Verification items for the finished model (mm, model axes). A direction names the side the tool comes from. Coordinates: 2 decimals unless noted, no trailing zeros. Write each loop counter-clockwise with the first axis right and the second up, starting at its lowest first coordinate (ties: lowest second). Pieces come first, ordered by that corner, then holes. Notation, with made-up numbers: M -39.5,44.25 L -34.5,44.25 A23 cw -34.5,67.25 Z; hole C 16.5,50 d5. An arc over 180 degrees is marked long. Answer in a Markdown table with one row per item.
from build123d import *

# Parameters (mm, degrees)
BOSS_EXTRUDE2_DEPTH = 3
CUT_EXTRUDE1_REACH  = 5
SKETCH2_R           = 1
SKETCH3_W           = 5.601007624
SKETCH3_H           = 10
BOSS_EXTRUDE3_DEPTH = 8
CHAMFER1_SIZE       = 1
CHAMFER1_SIZE2      = 2.747477419
CHAMFER2_SIZE       = 1
CHAMFER2_SIZE2      = 2.747477419
CHAMFER3_SIZE       = 1
CHAMFER3_SIZE2      = 2.747477419
CHAMFER4_SIZE       = 1
CHAMFER4_SIZE2      = 2.747477419
SKETCH4_W           = 7.688117752
SKETCH4_H           = 25
BOSS_EXTRUDE4_DEPTH = 8
SKETCH5_R           = 3.48412519
BOSS_EXTRUDE5_DEPTH = 9


with BuildPart() as part:
    # Sketch1 → Boss-Extrude2 (new body)
    with BuildSketch(Plane.XY):
        with BuildLine():
            Line((-10.7, 31.25), (10.7, 31.25))
            ThreePointArc((10.7, 31.25), (12.114213562, 30.664213562), (12.7, 29.25))
            Line((12.7, 29.25), (12.7, -29.25))
            ThreePointArc((12.7, -29.25), (12.114213562, -30.664213562), (10.7, -31.25))
            Line((10.7, -31.25), (-10.7, -31.25))
            ThreePointArc((-10.7, -31.25), (-12.114213562, -30.664213562), (-12.7, -29.25))
            Line((-12.7, -29.25), (-12.7, 29.25))
            ThreePointArc((-12.7, 29.25), (-12.114213562, 30.664213562), (-10.7, 31.25))
        make_face()
    extrude(amount=BOSS_EXTRUDE2_DEPTH)

    # Sketch2 → Cut-Extrude1 (cut, up to next)
    with BuildSketch(Plane.XY.offset(3), mode=Mode.PRIVATE) as cut_extrude1_sk1:
        with Locations((-10.7, 29.25)):
            Circle(SKETCH2_R)
    cut_extrude1_tool1 = extrude(cut_extrude1_sk1.sketch, amount=-CUT_EXTRUDE1_REACH, mode=Mode.PRIVATE) & part.part
    add(cut_extrude1_tool1.solids().sort_by_distance((-10.7, 29.25, 3))[0], mode=Mode.SUBTRACT)
    # Sketch2 → Cut-Extrude1 (cut, up to next)
    with BuildSketch(Plane.XY.offset(3), mode=Mode.PRIVATE) as cut_extrude1_sk2:
        with Locations((10.7, 29.25)):
            Circle(SKETCH2_R)
    cut_extrude1_tool2 = extrude(cut_extrude1_sk2.sketch, amount=-CUT_EXTRUDE1_REACH, mode=Mode.PRIVATE) & part.part
    add(cut_extrude1_tool2.solids().sort_by_distance((10.7, 29.25, 3))[0], mode=Mode.SUBTRACT)
    # Sketch2 → Cut-Extrude1 (cut, up to next)
    with BuildSketch(Plane.XY.offset(3), mode=Mode.PRIVATE) as cut_extrude1_sk3:
        with Locations((10.7, -29.25)):
            Circle(SKETCH2_R)
    cut_extrude1_tool3 = extrude(cut_extrude1_sk3.sketch, amount=-CUT_EXTRUDE1_REACH, mode=Mode.PRIVATE) & part.part
    add(cut_extrude1_tool3.solids().sort_by_distance((10.7, -29.25, 3))[0], mode=Mode.SUBTRACT)
    # Sketch2 → Cut-Extrude1 (cut, up to next)
    with BuildSketch(Plane.XY.offset(3), mode=Mode.PRIVATE) as cut_extrude1_sk4:
        with Locations((-10.7, -29.25)):
            Circle(SKETCH2_R)
    cut_extrude1_tool4 = extrude(cut_extrude1_sk4.sketch, amount=-CUT_EXTRUDE1_REACH, mode=Mode.PRIVATE) & part.part
    add(cut_extrude1_tool4.solids().sort_by_distance((-10.7, -29.25, 3))[0], mode=Mode.SUBTRACT)

    # Sketch3 → Boss-Extrude3 (add)
    with BuildSketch(Plane.XY.offset(3)):
        with Locations((-9.454083627, 0)):
            Rectangle(SKETCH3_W, SKETCH3_H)
    extrude(amount=BOSS_EXTRUDE3_DEPTH)

    # Chamfer1
    chamfer1_edges = [part.edges().sort_by_distance(p)[0] for p in [
        (-9.454083627, -5, 11),
    ]]
    chamfer1_side = [part.faces().sort_by_distance(p)[0] for p in [
        (-9.454083627, 0, 11),
    ]]
    chamfer(chamfer1_edges, length=CHAMFER1_SIZE, length2=CHAMFER1_SIZE2, reference=chamfer1_side[0])

    # Chamfer2
    chamfer2_edges = [part.edges().sort_by_distance(p)[0] for p in [
        (-9.454083627, 5, 11),
    ]]
    chamfer2_side = [part.faces().sort_by_distance(p)[0] for p in [
        (-9.454083627, 0.5, 11),
    ]]
    chamfer(chamfer2_edges, length=CHAMFER2_SIZE, length2=CHAMFER2_SIZE2, reference=chamfer2_side[0])

    # Chamfer3
    chamfer3_edges = [part.edges().sort_by_distance(p)[0] for p in [
        (-12.254587439, 0, 11),
    ]]
    chamfer3_side = [part.faces().sort_by_distance(p)[0] for p in [
        (-9.454083627, 0, 11),
    ]]
    chamfer(chamfer3_edges, length=CHAMFER3_SIZE, length2=CHAMFER3_SIZE2, reference=chamfer3_side[0])

    # Chamfer4
    chamfer4_edges = [part.edges().sort_by_distance(p)[0] for p in [
        (-6.653579815, 0, 11),
    ]]
    chamfer4_side = [part.faces().sort_by_distance(p)[0] for p in [
        (-8.954083627, 0, 11),
    ]]
    chamfer(chamfer4_edges, length=CHAMFER4_SIZE, length2=CHAMFER4_SIZE2, reference=chamfer4_side[0])

    # Sketch4 → Boss-Extrude4 (add)
    with BuildSketch(Plane.XY.offset(3)):
        with Locations((8.855941124, -14.499959716)):
            Rectangle(SKETCH4_W, SKETCH4_H)
        with Locations((8.855941124, 14.499959716)):
            Rectangle(SKETCH4_W, SKETCH4_H)
    extrude(amount=BOSS_EXTRUDE4_DEPTH)

    # Sketch5 → Boss-Extrude5 (add)
    with BuildSketch(Plane.XY.offset(3)):
        with Locations((-9.21587481, -21.073650693)):
            Circle(SKETCH5_R)
    extrude(amount=BOSS_EXTRUDE5_DEPTH)


solid = part.part
1) Tool access check on faces 4 (the face through (5.012, -15, 7)), 5 (the face through (9, 27, 7)), 6 (the face through (-11.76, -0.07, 9.61)). Record the directions out of +Z, -Z, +X, -X, +Y, -Y that give a thin tool (end or side, any length) a straight path to the whole face; none if there is none.
Response values:
| item | result |
|---|---|
| face 4 | +Z, +Y, -Y |
| face 5 | +Z, +X, -X, +Y |
| face 6 | +Z, -X, +Y |
2) Thickness scan on L1, parallel to Y at x = -10.7, z = 1.6; L2, parallel to Y at x = 7, z = 8.75; L3, parallel to Z at x = 3.25, y = -26.5. Record the ranges inside material, lowest first. Write a range as [from, to].
Response values:
| item | result |
|---|---|
| L1 | y = [-31.25, -30.25], [-28.25, 28.25], [30.25, 31.25] |
| L2 | y = [-27, -2], [2, 27] |
| L3 | z = [0, 3] |
3) Depth check by flat-ended pin: pin 1 (1.5 mm diameter, centred on y = -24, z = 8.5, fed in from -X); pin 2 (4 mm diameter, centred on x = 8, y = -18, fed in from +Z); pin 3 (6.5 mm diameter, centred on y = -11.5, z = 8, fed in from -X); pin 4 (1.8 mm diameter, centred on x = 10.7, y = -29.25, fed in from -Z). Enter the tip coordinate at first touch or a pass-through.
Response values:
| item | result |
|---|---|
| pin 1 | stops at x = -11.94 |
| pin 2 | stops at z = 11 |
| pin 3 | stops at x = 5.01 |
| pin 4 | passes through |
4) Sectioned sample at D-D (x = 3.75). Record the cut outline in (y, z).
Response values:
| item | result |
|---|---|
| outline | M -31.25,0 L 31.25,0 L 31.25,3 L -31.25,3 Z |
5) Sectioned sample at C-C (y = -12.5). Record the cut outline in (x, z), then the cut area to 3 significant figures.
Response values:
| item | result |
|---|---|
| outline | M -12.7,0 L 12.7,0 L 12.7,11 L 5.01,11 L 5.01,3 L -12.7,3 Z |
| area | 138 mm² |
6) Sectioned sample at A-A (z = 7.5). Record the cut outline in (x, y), then the cut area to 3 significant figures.
Response values:
| item | result |
|---|---|
| outline | C -9.22,-21.07 d6.97; M -12.25,-5 L -6.65,-5 L -6.65,5 L -12.25,5 Z; M 5.01,-27 L 12.7,-27 L 12.7,-2 L 5.01,-2 Z; M 5.01,2 L 12.7,2 L 12.7,27 L 5.01,27 Z |
| area | 479 mm² |
7) Sectioned sample at B-B (x = 6.75). Record the cut outline in (y, z), then the cut area to 4 significant figures.
Response values:
| item | result |
|---|---|
| outline | M -31.25,0 L 31.25,0 L 31.25,3 L 27,3 L 27,11 L 2,11 L 2,3 L -2,3 L -2,11 L -27,11 L -27,3 L -31.25,3 Z |
| area | 587.5 mm² |
8) Release check for a two-part mould opening along X. For faces 1 (the face through (12.7, 0, 2)), 2 (the face through (0, 0, 0)), 3 (the face through (-6.654, 0, 6)) record: +X half, -X half, draft (parallel to the pull), parting line (faces both ways), or undercut.
Response values:
| item | result |
|---|---|
| face 1 | +X half |
| face 2 | draft |
| face 3 | undercut |
